Geometry: final body of the model. Coordinates: model frame, mm. A direction names the side the tool comes from. Give positions to 0.01 mm unless a question says otherwise; leave off trailing zeros. Write each loop counter-clockwise with the first axis right and the second up, starting at its lowest first coordinate (ties: lowest second). Pieces come first, ordered by that corner, then holes. Notation, with made-up numbers: M 29,58.5 L 78,58.5 A16 ccw 78,72.5 Z; hole C 28.5,14 d2. An arc over 180 degrees is marked long. Use one line per item in the form item = value. Start each with the question number.
Item 1: Section query A-A on x = -2. Return loops of the section in (y, z).
Item 2: Material intervals for line 1 along X through (y, z) = (4.8, -45); line 2 along Z through (x, y) = (36, 44); line 3 along X through (y, z) = (-0.55, -45), sorted ascending. Write a range as from..to.
Item 3: Section query D-D on z = 27.5. Return loops of the section in (x, y).
Item 4: Pull-direction query (Z, two-part tool) for faces 1 (the flat face through (1, 56, -60.86)), 2 (the cylindrical face through (26.62, 4.48, -45.51)), 3 (the cylindrical face through (-38.924, 106.993, 56.412)); classes: released by +Z, released by -Z, zero draft, split by the parting line, or undercut.
Item 5: Section query C-C on z = -45. Give the number of separate pieces and of enclosed holes in the cut face, then the cut area to 3 significant figures.
Item 6: Access query for faces 4 (the flat face through (0.529, 16.985, 3.39)), 5 (the cylindrical face through (-33.65, 106.99, -60.42)), 6 (the flat face through (0.53, 17.39, 1.57)), 7 (the cylindrical face through (35.65, 106.99, 60.42)). Directions: +Z, -Z, +X, -X, +Y, -Y. A direction counts if a zero-diameter tool reaches every point of the face in a straight line with its end or side. Return the directions, or none.
Item 7: Contact query for flat-ended pins moving along their axis: P1, Ø2, axis at x = -25, z = -45, coming from the +Y side; P2, Ø0.8, axis at y = 67.5, z = 60.5, coming from the -X side; P3, Ø1.8, axis at x = -38.5, y = 40, coming from the -Z side; P4, Ø5, axis at x = -4, z = 43, coming from the +Y side. Output: stop coordinate, or through.
Item 8: Section query B-B on y = 74. Return loops of the section in (x, z).
from build123d import *

# Parameters (mm, degrees)
SKETCH1_W                    = 77
SKETCH1_H                    = 120
BASE_FLANGE1_DEPTH           = 0.86
EDGE_FLANGE1_STRIP_W         = 4.9132
EDGE_FLANGE1_STRIP_H         = 0.86
EDGE_FLANGE1_STRIP_CUT_DEPTH = 77
EDGE_FLANGE1_DEPTH           = 77
EDGE_FLANGE2_STRIP_W         = 4.9132
EDGE_FLANGE2_STRIP_H         = 0.86
EDGE_FLANGE2_STRIP_CUT_DEPTH = 119.2634
EDGE_FLANGE2_DEPTH           = 119.2634
EDGE_FLANGE3_STRIP_W         = 4.9132
EDGE_FLANGE3_STRIP_H         = 0.86
EDGE_FLANGE3_STRIP_CUT_DEPTH = 119.2634
EDGE_FLANGE3_DEPTH           = 119.2634
EDGE_FLANGE4_STRIP_CUT_DEPTH = 75.5268
EDGE_FLANGE4_DEPTH           = 75.5268
EDGE_FLANGE8_STRIP_W         = 4.9132
EDGE_FLANGE8_STRIP_H         = 0.86
EDGE_FLANGE8_STRIP_CUT_DEPTH = 109.2634
EDGE_FLANGE8_DEPTH           = 109.2634
M3_CLEARANCE_HOLE3_D         = 3.4
M3_CLEARANCE_HOLE3_DEPTH     = 25.4
M3_CLEARANCE_HOLE3_TIP       = 1.021463052
FILLET1_R                    = 10


# Sheet-metal steps are written as plain solids
with BuildPart() as part:
    # Sketch1 → Base-Flange1 (new body)
    with BuildSketch(Plane(origin=(0, 0, 0), x_dir=(1, 0, 0), z_dir=(0, 1, 0))):
        Rectangle(SKETCH1_W, SKETCH1_H)
    extrude(amount=-BASE_FLANGE1_DEPTH)

    # Edge-Flange1 strip (across the edge) → Edge-Flange1 strip cut (cut)
    with BuildSketch(Plane(origin=(-38.5, 0, 60), x_dir=(0, 0, -1), z_dir=(1, 0, 0))):
        with Locations((-1.72, -0.43)):
            Rectangle(EDGE_FLANGE1_STRIP_W, EDGE_FLANGE1_STRIP_H)
    extrude(amount=EDGE_FLANGE1_STRIP_CUT_DEPTH, mode=Mode.SUBTRACT)

    # Edge-Flange1 section (across the edge) → Edge-Flange1 (add)
    with BuildSketch(Plane(origin=(-38.5, 0, 60), x_dir=(0, 0, -1), z_dir=(1, 0, 0))):
        with BuildLine():
            Line((-0.86, 0.7366), (-0.86, 110))
            Line((-0.86, 110), (0, 110))
            Line((0, 110), (0, 0.7366))
            ThreePointArc((0, 0.7366), (0.215745145, 0.215745145), (0.7366, 0))
            Line((0.7366, 0), (0.7366, -0.86))
            ThreePointArc((0.7366, -0.86), (-0.392366687, -0.392366687), (-0.86, 0.7366))
        make_face()
    extrude(amount=EDGE_FLANGE1_DEPTH)

    # Edge-Flange2 strip (across the edge) → Edge-Flange2 strip cut (cut)
    with BuildSketch(Plane(origin=(38.5, 0, 59.2634), x_dir=(-1, 0, 0), z_dir=(0, 0, -1))):
        with Locations((-1.72, -0.43)):
            Rectangle(EDGE_FLANGE2_STRIP_W, EDGE_FLANGE2_STRIP_H)
    extrude(amount=EDGE_FLANGE2_STRIP_CUT_DEPTH, mode=Mode.SUBTRACT)

    # Edge-Flange2 section (across the edge) → Edge-Flange2 (add)
    with BuildSketch(Plane(origin=(38.5, 0, 59.2634), x_dir=(-1, 0, 0), z_dir=(0, 0, -1))):
        with BuildLine():
            Line((-0.86, 0.7366), (-0.86, 110))
            Line((-0.86, 110), (0, 110))
            Line((0, 110), (0, 0.7366))
            ThreePointArc((0, 0.7366), (0.215745145, 0.215745145), (0.7366, 0))
            Line((0.7366, 0), (0.7366, -0.86))
            ThreePointArc((0.7366, -0.86), (-0.392366687, -0.392366687), (-0.86, 0.7366))
        make_face()
    extrude(amount=EDGE_FLANGE2_DEPTH)

    # Edge-Flange3 strip (across the edge) → Edge-Flange3 strip cut (cut)
    with BuildSketch(Plane(origin=(-38.5, 0, -60), x_dir=(1, 0, 0), z_dir=(0, 0, 1))):
        with Locations((-1.72, -0.43)):
            Rectangle(EDGE_FLANGE3_STRIP_W, EDGE_FLANGE3_STRIP_H)
    extrude(amount=EDGE_FLANGE3_STRIP_CUT_DEPTH, mode=Mode.SUBTRACT)

    # Edge-Flange3 section (across the edge) → Edge-Flange3 (add)
    with BuildSketch(Plane(origin=(-38.5, 0, -60), x_dir=(1, 0, 0), z_dir=(0, 0, 1))):
        with BuildLine():
            Line((-0.86, 0.7366), (-0.86, 110))
            Line((-0.86, 110), (0, 110))
            Line((0, 110), (0, 0.7366))
            ThreePointArc((0, 0.7366), (0.215745145, 0.215745145), (0.7366, 0))
            Line((0.7366, 0), (0.7366, -0.86))
            ThreePointArc((0.7366, -0.86), (-0.392366687, -0.392366687), (-0.86, 0.7366))
        make_face()
    extrude(amount=EDGE_FLANGE3_DEPTH)

    # Edge-Flange4 strip (across the edge) → Edge-Flange4 strip cut (cut)
    with BuildSketch(Plane(origin=(37.7634, 0, -60), x_dir=(0, -0.9659258262890681, 0.25881904510252135), z_dir=(-1, 0, 0))):
        Polygon((-7.380189595, -30.866027382), (2.278797174, 5.181801992), (1.448100964, 5.404386371), (-8.210885806, -30.643443003), align=None)
    extrude(amount=EDGE_FLANGE4_STRIP_CUT_DEPTH, mode=Mode.SUBTRACT)

    # Edge-Flange4 section (across the edge) → Edge-Flange4 (add)
    with BuildSketch(Plane(origin=(37.7634, 0, -60), x_dir=(0, -0.9659258262890681, 0.25881904510252135), z_dir=(-1, 0, 0))):
        with BuildLine():
            Line((-0.86, 5.595032479), (-0.86, 124))
            Line((-0.86, 124), (0, 124))
            Line((0, 124), (0, 5.595032479))
            ThreePointArc((0, 5.595032479), (0.640454407, 4.864734195), (1.448100964, 5.404386371))
            Line((1.448100964, 5.404386371), (2.278797174, 5.181801992))
            ThreePointArc((2.278797174, 5.181801992), (0.528201882, 4.012091614), (-0.86, 5.595032479))
        make_face()
    extrude(amount=EDGE_FLANGE4_DEPTH)

    # Edge-Flange8 strip (across the edge) → Edge-Flange8 strip cut (cut)
    with BuildSketch(Plane(origin=(38.5, 110, -60), x_dir=(0, 0, 1), z_dir=(0, -1, 0))):
        with Locations((-1.72, -0.43)):
            Rectangle(EDGE_FLANGE8_STRIP_W, EDGE_FLANGE8_STRIP_H)
    extrude(amount=EDGE_FLANGE8_STRIP_CUT_DEPTH, mode=Mode.SUBTRACT)

    # Edge-Flange8 section (across the edge) → Edge-Flange8 (add)
    with BuildSketch(Plane(origin=(38.5, 110, -60), x_dir=(0, 0, 1), z_dir=(0, -1, 0))):
        with BuildLine():
            Line((-0.86, 0.7366), (-0.86, 75))
            Line((-0.86, 75), (0, 75))
            Line((0, 75), (0, 0.7366))
            ThreePointArc((0, 0.7366), (0.215745145, 0.215745145), (0.7366, 0))
            Line((0.7366, 0), (0.7366, -0.86))
            ThreePointArc((0.7366, -0.86), (-0.392366687, -0.392366687), (-0.86, 0.7366))
        make_face()
    extrude(amount=EDGE_FLANGE8_DEPTH)

    # M3 Clearance Hole3
    with Locations(Plane(origin=(0, -0.86, 0), x_dir=(-1, 0, 0), z_dir=(0, -1, 0))):
        with Locations((-25, 45), (25, 45), (25, -45), (-25, -45)):
            Hole(M3_CLEARANCE_HOLE3_D / 2, depth=M3_CLEARANCE_HOLE3_DEPTH)
            with Locations((0, 0, -(M3_CLEARANCE_HOLE3_DEPTH + M3_CLEARANCE_HOLE3_TIP / 2))):  # 118° drill point
                Cone(0, M3_CLEARANCE_HOLE3_D / 2, M3_CLEARANCE_HOLE3_TIP, mode=Mode.SUBTRACT)

    # Fillet1
    fillet1_edges = [part.edges().sort_by_distance(p)[0] for p in [
        (-36.5, 0.7366, -60.43),
        (-36.5, 110, -60.43),
        (-38.93, 110, -60),
        (-38.93, 110, 59.2634),
        (38.93, 110, 59.2634),
        (38.5, 110, 60.43),
        (-38.5, 110, 60.43),
    ]]
    fillet(fillet1_edges, radius=FILLET1_R)


solid = part.part
Answer sheet:
q1.outline = M -0.86,-54.4 A1.6 ccw 2.28,-54.82 L 32.92,59.55 L 32.09,59.77 L 1.45,-54.6 A0.74 cw 0,-54.4 L 0,59.26 A0.74 cw 0.74,60 L 110,60 L 110,60.86 L 0.74,60.86 A1.6 ccw -0.86,59.26 Z; M 0.74,-60.86 L 110,-60.86 L 110,-60 L 0.74,-60 Z
q2.line_1 = -39.36..-38.5, -37.76..-26.7, -23.3..23.3, 26.7..37.76, 38.5..39.36
q2.line_2 = -60.86..-60, 60..60.86
q2.line_3 = -38.71..-26.7, -23.3..23.3, 26.7..38.71
q3.outline = M -39.36,0.74 A1.6 ccw -37.76,-0.86 L 37.76,-0.86 A1.6 ccw 39.36,0.74 L 39.36,110 L 38.5,110 L 38.5,0.74 A0.74 cw 37.76,0 L -37.76,0 A0.74 cw -38.5,0.74 L -38.5,110 L -39.36,110 Z; M -37.76,23.45 L 37.76,23.45 L 37.76,24.34 L -37.76,24.34 Z
q4.face_1 = released by -Z
q4.face_2 = undercut
q4.face_3 = released by +Z
q5.separate_pieces = 6
q5.enclosed_holes = 0
q5.area = 311 mm2
q6.face_4 = none
q6.face_5 = -Z, -X, +Y
q6.face_6 = +Y
q6.face_7 = +Z, +X, +Y
q7.P1 = through
q7.P2 = -38.5
q7.P3 = -60
q7.P4 = 29.16
q8.outline = M -39.36,-60 L -38.5,-60 L -38.5,59.26 L -39.36,59.26 Z; M -38.5,60 L 38.5,60 L 38.5,60.86 L -38.5,60.86 Z; M -36.5,-60.86 L 37.76,-60.86 A1.6 ccw 39.36,-59.26 L 39.36,59.26 L 38.5,59.26 L 38.5,-59.26 A0.74 cw 37.76,-60 L -36.5,-60 Z
